The model under review builds one solid part; all positions refer to its coordinate system, in mm. A direction names the side the tool comes from. Round coordinates to 2 decimals unless told otherwise and drop trailing zeros. Order: outer loops, then holes, each group sorted by start corner. A loop starts at its lowest first (then second) coordinate and runs counter-clockwise, first axis right, second up. Notation, with made-up numbers: M 64,69.25 L 68,69.25 A15 ccw 68,74.25 Z; hole C -3.75,-10 d4. An arc over 180 degrees is marked long. Use a Markdown table: item, result. Add a question column.
1. Consider section A-A on y = 0. State the section outline as (x, z) points.
2. Consider section B-B on x = 8.5. State the section outline as (y, z) points.
3. For faces 4 (the flat face through (127, 0, 3)), 5 (the cylindrical face through (-18.03, 0.4, 2.58)), list the 3-axis set-ups (+Z, -Z, +X, -X, +Y, -Y) from which the entire face can be reached by the end or side of a thin tool; tool diameter is ignored.
4. The part is to be moulded in two halves that separate along X. For faces 1 (the flat face through (19, -18.034, 3)), 2 (the flat face through (63, -19.939, 3)), 3 (the cylindrical face through (-19.934, 0.438, 2.504)), say which applies: +X half, -X half, draft (parallel to the pull), parting line (faces both ways), or undercut.
5. To check wall thickness, follow probe 1 along Y at (x, z) = (8, 2.5); probe 2 along X at (y, z) = (0, 4.3); probe 3 along X at (y, z) = (-4, 1.6). State the ranges of each line that lie inside material, in increasing order.
6. Insertion check: P1, Ø3, axis at y = 10.5, z = 2, coming from the -X side; P2, Ø2, axis at y = -12, z = 2, coming from the -X side. Each pin has a flat end and moves straight along its axis. Give the tip position at first contact, or say it passes through.
from build123d import *

# Parameters (mm, degrees)
SKETCH1_R               = 19.939
CIRCLE_EXTRUDE_DEPTH    = 5.08
SKETCH3_W               = 5.08
SKETCH3_H               = 39.878
RECTANGLE_EXTRUDE_DEPTH = 127
SKETCH2_R               = 18.034
CIRCLE_CUT_DEPTH        = 129.65601471
SKETCH6_W               = 125.095
SKETCH6_H               = 36.068
RECTANGLE_CUT_DEPTH     = 129.65601471
END_SHAPE_DEPTH         = 5.08


with BuildPart() as part:
    # Sketch1 → circle extrude (new body)
    with BuildSketch(Plane.XY):
        Circle(SKETCH1_R)
    extrude(amount=CIRCLE_EXTRUDE_DEPTH)

    # Sketch3 → rectangle extrude (add)
    with BuildSketch(Plane(origin=(0, 0, 0), x_dir=(0, 0, -1), z_dir=(1, 0, 0))):
        with Locations((-2.54, 0)):
            Rectangle(SKETCH3_W, SKETCH3_H)
    extrude(amount=RECTANGLE_EXTRUDE_DEPTH)

    # Sketch2 → circle cut (cut, through all)
    with BuildSketch(Plane.XY.offset(5.08)):
        Circle(SKETCH2_R)
    extrude(amount=-CIRCLE_CUT_DEPTH, mode=Mode.SUBTRACT)

    # Sketch6 → rectangle cut (cut, through all)
    with BuildSketch(Plane.XY.offset(5.08)):
        with Locations((62.5475, 0)):
            Rectangle(SKETCH6_W, SKETCH6_H)
    extrude(amount=-RECTANGLE_CUT_DEPTH, mode=Mode.SUBTRACT)

    # Sketch7 → end shape (add)
    with BuildSketch(Plane.XY.offset(5.08)):
        with BuildLine():
            Line((38.354, 18.034), (125.095, 18.034))
            Line((125.095, 18.034), (125.095, -18.034))
            Line((125.095, -18.034), (38.354, -18.034))
            ThreePointArc((38.354, -18.034), (56.388, 0), (38.354, 18.034))
        make_face()
    extrude(amount=-END_SHAPE_DEPTH)


solid = part.part
Answer block:
| question | item | result |
|---|---|---|
| 1 | outline | M -19.94,0 L -18.03,0 L -18.03,5.08 L -19.94,5.08 Z; M 56.39,0 L 127,0 L 127,5.08 L 56.39,5.08 Z |
| 2 | outline | M -19.94,0 L -18.03,0 L -18.03,5.08 L -19.94,5.08 Z; M 18.03,0 L 19.94,0 L 19.94,5.08 L 18.03,5.08 Z |
| 3 | face 4 | +Z, -Z, +X, +Y, -Y |
| 3 | face 5 | +Z, -Z |
| 4 | face 1 | undercut |
| 4 | face 2 | draft |
| 4 | face 3 | -X half |
| 5 | probe 1 | -19.94 to -18.03, 18.03 to 19.94 |
| 5 | probe 2 | -19.94 to -18.03, 56.39 to 127 |
| 5 | probe 3 | -19.53 to -17.58, 55.94 to 127 |
| 6 | P1 | x = -17.79 |
| 6 | P2 | x = -16.63 |
